```python
from build123d import *

# Parameters (mm, degrees)
SKETCH1_R           = 2.72
BOSS_EXTRUDE1_DEPTH = 3
SKETCH2_R           = 1.44
BOSS_EXTRUDE2_DEPTH = 8
CUT_EXTRUDE1_DEPTH  = 1.95
FILLET1_R           = 0.5


with BuildPart() as part:
    # Sketch1 → Boss-Extrude1 (new body)
    with BuildSketch(Plane(origin=(0, 0, 0), x_dir=(1, 0, 0), z_dir=(0, 1, 0))):
        Circle(SKETCH1_R)
    extrude(amount=BOSS_EXTRUDE1_DEPTH)

    # Sketch2 → Boss-Extrude2 (add)
    with BuildSketch(Plane.XZ):
        Circle(SKETCH2_R)
    extrude(amount=BOSS_EXTRUDE2_DEPTH)

    # Sketch3 → Cut-Extrude1 (cut)
    with BuildSketch(Plane(origin=(0, 3, 0), x_dir=(1, 0, 0), z_dir=(0, 1, 0))):
        Polygon((1.10418239, 0.6375), (0, 1.275), (-1.10418239, 0.6375), (-1.10418239, -0.6375), (0, -1.275), (1.10418239, -0.6375), align=None)
    extrude(amount=-CUT_EXTRUDE1_DEPTH, mode=Mode.SUBTRACT)

    # Fillet1
    fillet1_edges = [part.edges().sort_by_distance(p)[0] for p in [
        (-2.72, 3, 0),
    ]]
    fillet(fillet1_edges, radius=FILLET1_R)


solid = part.part
```
For this review, take the finished solid that the model builds, in its own axes (mm). A direction names the side the tool comes from. Round coordinates to 2 decimals unless told otherwise and drop trailing zeros. Loops run counter-clockwise (first coordinate to the right, second up) from the corner with the lowest first, then second, coordinate; pieces in that order, holes last.
Q1. Add section A-A on z = 0. Write out the cut boundary in (x, y).
Result sheet:
outline: (-2.72, 0) - (-1.44, 0) - (-1.44, -8) - (1.44, -8) - (1.44, 0) - (2.72, 0) - (2.72, 2.5) arc R0.5 ccw to (2.22, 3) - (1.1, 3) - (1.1, 1.05) - (-1.1, 1.05) - (-1.1, 3) - (-2.22, 3) arc R0.5 ccw to (-2.72, 2.5) - close
Q2. Machinability: for faces 4 (the face through (0, -8, 0)), 5 (the face through (0, 1.05, 0)), 6 (the face through (1.2, 0, 1.2)), which of the approach directions +Z, -Z, +X, -X, +Y, -Y give a long, thin tool a straight path to every point of the face, cutting with its end or side? Answer none if there is none.
Result sheet:
face 4: +Z, -Z, +X, -X, -Y
face 5: +Y
face 6: -Y
Q3. Mouldability with a two-part tool opening along X and no side actions: class faces 1 (the face through (-0.56, 2.04, 0.95)), 2 (the face through (-1, 3, -1)), 3 (the face through (2.6, 1.2, -0.8)) as +X half, -X half, draft (parallel to the pull), parting line (faces both ways), or undercut.
Result sheet:
face 1: undercut
face 2: draft
face 3: parting line
Q4. To check wall thickness, follow line 1 along Z through (x, y) = (0, -1.25); line 2 along Y through (x, z) = (-0.3, -2.1); line 3 along Y through (x, z) = (0.35, 0.05). State the ranges of each line that lie inside material, in increasing order.
Result sheet:
line 1: z = -1.44 to 1.44
line 2: y = 0 to 3
line 3: y = -8 to 1.05
Q5. Insertion check: pin 1 Ø3 at (y, z) = (0.5, 1) entering from +X. The pin has a flat end and moves straight along its axis. Give the tip position at first contact, or say it passes through.
Result sheet:
pin 1: stops at x = 2.72
Q6. Add section B-B on y = -0.75. Write out the cut boundary in (x, z).
Result sheet:
outline: circle Ø2.88 at (0, 0)
